Work out the finished part from the listing and answer in its coordinate system (mm). Coordinates: 2 decimals unless noted, no trailing zeros. Write each loop counter-clockwise with the first axis right and the second up, starting at its lowest first coordinate (ties: lowest second). Pieces come first, ordered by that corner, then holes. Notation, with made-up numbers: (-32, 65.25) - (-20, 65.25) arc R25 cw to (-20, 96.25) - close; hole circle Ø8 at (-9.75, -4). An arc over 180 degrees is marked (long way). Use one line per item in the form item = value. Start each with the question number.
Item 1: A cutting plane is placed at B-B (x = -0.25). Give the number of separate pieces and of enclosed holes in the cut face, then the cut area to 3 significant figures.
Item 2: Determine the mould class of faces 1 (the cylindrical face through (0.65, 1.37, 87.07)), 2 (the flat face through (0, 0, 117.5)), 3 (the flat face through (0, 3.25, -2)) for opening direction Z: released by +Z, released by -Z, zero draft, split by the parting line, or undercut.
Item 3: Consider probe 1 along X at (y, z) = (1.5, -1.5); probe 2 along Y at (x, z) = (3.5, 107.5); probe 3 along X at (y, z) = (0.5, -23). Determine where each line is inside the solid, lowest interval first.
Item 4: Given pin 1 (5 mm diameter, centred on x = 0, z = -70, fed in from +Y); pin 2 (5 mm diameter, centred on x = -0.5, z = -111.5, fed in from +Y); pin 3 (4 mm diameter, centred on x = 0, z = -10, fed in from -Y), each flat-ended and moving along its own axis, determine where each tip first touches the part or whether it passes through.
Item 5: A cutting plane is placed at A-A (z = 79.5). Write down the section's boundary in (x, y).
Autodesk Inventor part; units mm, degrees
ref_plane "to_body_XY" through (0, -3.25, 0) normal (0, 0, 1) x (1, 0, 0)
ref_plane "to_body_YZ" through (0, -3.25, 0) normal (1, 0, 0) x (0, 1, 0)
ref_plane "to_body_ZX" through (0, -3.25, 0) normal (0, 1, 0) x (0, 0, 1)
sketch "_____1" plane through (0, 0, 0) normal (0, 0, 1) x (1, 0, 0)
  line L0 (-4.5, 2.95) -> (-4.5, 2.1665)
  arc A0 (-3.9835, 1.65) -> (-4.5, 2.1665) centre (-4.9, 1.25) ccw
  line L1 (-3.9835, 1.65) -> (-3.6, 1.65)
  arc A1 (-3.6, 0.85) -> (-3.6, 1.65) centre (-3.6, 1.25) ccw
  line L2 (-3.6, 0.85) -> (-3.9835, 0.85)
  arc A2 (-4.5, 0.3335) -> (-3.9835, 0.85) centre (-4.9, 1.25) ccw
  line L3 (-4.5, 0.3335) -> (-4.5, -2.95)
  line L4 (-4.5, -2.95) -> (-4.2, -3.25)
  line L5 (-4.2, -3.25) -> (4.2, -3.25)
  line L6 (4.2, -3.25) -> (4.5, -2.95)
  line L7 (4.5, -2.95) -> (4.5, 0.3335)
  arc A3 (3.9835, 0.85) -> (4.5, 0.3335) centre (4.9, 1.25) ccw
  line L8 (3.9835, 0.85) -> (3.6, 0.85)
  arc A4 (3.6, 1.65) -> (3.6, 0.85) centre (3.6, 1.25) ccw
  line L9 (3.6, 1.65) -> (3.9835, 1.65)
  arc A5 (4.5, 2.1665) -> (3.9835, 1.65) centre (4.9, 1.25) ccw
  line L10 (4.5, 2.1665) -> (4.5, 2.95)
  line L11 (4.5, 2.95) -> (4.2, 3.25)
  line L12 (4.2, 3.25) -> (-4.2, 3.25)
  line L13 (-4.2, 3.25) -> (-4.5, 2.95)
extrude "Extrusion1" add sketch "_____1" along normal mid plane 235
sketch "_____5" plane through (0, 0, 110) normal (0, 0, 1) x (1, 0, 0)
  line L0 (0, 3.25) -> (0, -3.25)
  line L1 (0, -3.25) -> (-2.05, -3.25)
  line L2 (-2.05, -3.25) -> (-1.75, -2.95)
  line L3 (-1.75, -2.95) -> (-1.75, -0.25)
  line L4 (-1.75, -0.25) -> (-3, -0.25)
  line L5 (-3, -0.25) -> (-3, 2.95)
  line L6 (-3, 2.95) -> (-3.3, 3.25)
  line L7 (-3.3, 3.25) -> (0, 3.25)
  line L8 (0, 3.25) -> (0, -3.25)
revolve "Revolution1" cut sketch "_____5" angle 360 about axis through (0, 3.25, 110) along (0, 1, 0)
pattern_linear "Rectangular Pattern1" count 12 spacing 20 along (0, 0, -1) of "Revolution1"
ref_plane "to_body_XY" through (0, -3.25, 0) normal (0, 0, 1) x (1, 0, 0)
ref_plane "to_body_YZ" through (0, -3.25, 0) normal (1, 0, 0) x (0, 1, 0)
ref_plane "to_body_ZX" through (0, -3.25, 0) normal (0, 1, 0) x (0, 0, 1)
properties part number "C-MLG9-235_r"
Answer:
q1.separate_pieces = 13
q1.enclosed_holes = 0
q1.area = 1,150 mm²
q2.face_1 = undercut
q2.face_2 = released by +Z
q2.face_3 = zero draft
q3.probe_1 = -3.29 to 3.29
q3.probe_2 = -3.25 to 0.86, 1.64 to 3.25
q3.probe_3 = -4.24 to 4.24
q4.pin_1 = -0.25
q4.pin_2 = 3.25
q4.pin_3 = -3.2
q5.outline = (-4.5, -2.95) - (-4.2, -3.25) - (4.2, -3.25) - (4.5, -2.95) - (4.5, 0.33) arc R1 cw to (3.98, 0.85) - (3.6, 0.85) arc R0.4 cw to (3.6, 1.65) - (3.98, 1.65) arc R1 cw to (4.5, 2.17) - (4.5, 2.95) - (4.2, 3.25) - (-4.2, 3.25) - (-4.5, 2.95) - (-4.5, 2.17) arc R1 cw to (-3.98, 1.65) - (-3.6, 1.65) arc R0.4 cw to (-3.6, 0.85) - (-3.98, 0.85) arc R1 cw to (-4.5, 0.33) - close
